Work out the finished part from the listing and answer in its coordinate system (mm). Face numbers are marked on the shaded views. A direction names the side the tool comes from. Round coordinates to 2 decimals unless told otherwise and drop trailing zeros. Write each loop counter-clockwise with the first axis right and the second up, starting at its lowest first coordinate (ties: lowest second). Pieces come first, ordered by that corner, then holes. Notation, with made-up numbers: (80, 82) - (105, 82) arc R25 cw to (105, 119) - close; hole circle Ø7 at (-16.5, 29). An arc over 180 degrees is marked (long way). Answer as a JSON object with one key per item and string values.
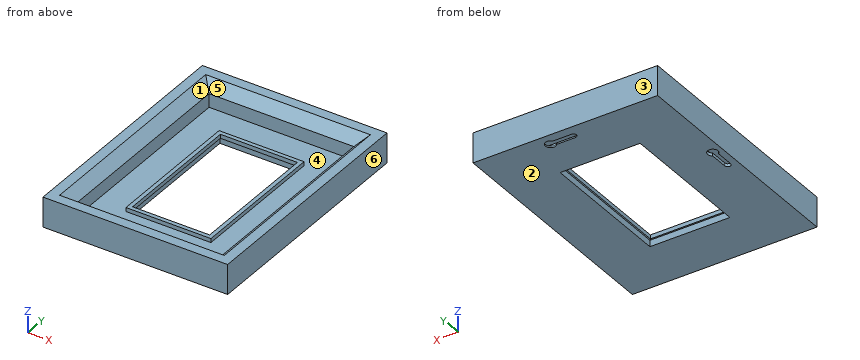
```python
from build123d import *

# Parameters (mm, degrees)
SKETCH_W             = 185.32
SKETCH_H             = 240.5
PAD_DEPTH            = 30
SKETCH003_W          = 145.32
SKETCH003_H          = 200.5
POCKET_DEPTH         = 23.6
SKETCH004_W          = 80.32
SKETCH004_H          = 135.5
POCKET001_DEPTH      = 6.4
POCKET002_DEPTH      = 3
SKETCH006_W          = 14
SKETCH006_H          = 3
POCKET003_DEPTH      = 30
POCKET004_DEPTH      = 1.5
SKETCH008_W          = 12
SKETCH008_H          = 2.4244
POCKET005_DEPTH      = 30
SKETCH009_W          = 85.32
SKETCH009_H          = 140.5
PAD001_DEPTH         = 4
SKETCH010_W          = 77.32
SKETCH010_H          = 132.5
POCKET006_DEPTH      = 0.001
POCKET006_DEPTH_BACK = -30.001
CHAMFER_SIZE         = 10


with BuildPart() as part:
    # Sketch → Pad (new body)
    with BuildSketch(Plane.XY):
        Rectangle(SKETCH_W, SKETCH_H)
    extrude(amount=PAD_DEPTH)

    # Sketch003 → Pocket (cut)
    with BuildSketch(Plane.XY.offset(30)):
        Rectangle(SKETCH003_W, SKETCH003_H)
    extrude(amount=-POCKET_DEPTH, mode=Mode.SUBTRACT)

    # Sketch004 → Pocket001 (cut)
    with BuildSketch(Plane.XY.offset(6.4)):
        Rectangle(SKETCH004_W, SKETCH004_H)
    extrude(amount=-POCKET001_DEPTH, mode=Mode.SUBTRACT)

    # Sketch005 → Pocket002 (cut)
    with BuildSketch(Plane.XY):
        with BuildLine():
            ThreePointArc((-85.97, 0), (-82.985, -2.985), (-80, 0))
            Line((-80, 0), (-80, 18.025988))
            ThreePointArc((-80, 18.025988), (-82.985, 27.495), (-85.97, 18.025988))
            Line((-85.97, 18.025988), (-85.97, 0))
        make_face()
    extrude(amount=POCKET002_DEPTH, mode=Mode.SUBTRACT)

    # Sketch006 → Pocket003 (cut, symmetric)
    with BuildSketch(Plane.XZ):
        with Locations((-83, 4.48)):
            Rectangle(SKETCH006_W, SKETCH006_H)
    extrude(amount=POCKET003_DEPTH, both=True, mode=Mode.SUBTRACT)

    # Sketch007 → Pocket004 (cut, symmetric)
    with BuildSketch(Plane.XY):
        with BuildLine():
            ThreePointArc((0, 110.985), (-2.985, 108), (0, 105.015))
            Line((0, 105.015), (18.705988, 105.015))
            ThreePointArc((18.705988, 105.015), (28.175, 108), (18.705988, 110.985))
            Line((18.705988, 110.985), (0, 110.985))
        make_face()
    extrude(amount=POCKET004_DEPTH, both=True, mode=Mode.SUBTRACT)

    # Sketch008 → Pocket005 (cut, symmetric)
    with BuildSketch(Plane.YZ):
        with Locations((108, 2.7105)):
            Rectangle(SKETCH008_W, SKETCH008_H)
    extrude(amount=POCKET005_DEPTH, both=True, mode=Mode.SUBTRACT)

    # Sketch009 → Pad001 (join)
    with BuildSketch(Plane.XY.offset(6.4)):
        Rectangle(SKETCH009_W, SKETCH009_H)
    extrude(amount=PAD001_DEPTH)

    # Sketch010 → Pocket006 (cut, two sides)
    with BuildSketch(Plane.XY) as pocket006_sk:
        Rectangle(SKETCH010_W, SKETCH010_H)
    extrude(amount=-POCKET006_DEPTH, mode=Mode.SUBTRACT)
    extrude(pocket006_sk.sketch, amount=-POCKET006_DEPTH_BACK, mode=Mode.SUBTRACT)

    # Chamfer
    chamfer_edges = [part.edges().sort_by_distance(p)[0] for p in [
        (-72.66, 0, 30),
        (0, 100.25, 30),
        (72.66, 0, 30),
        (0, -100.25, 30),
    ]]
    chamfer(chamfer_edges, length=CHAMFER_SIZE)


solid = part.part
```
Item 1: A cutting plane is placed at D-D (z = 26). Write down the section's boundary in (x, y).
Results found:
{"outline": "(-92.66, -120.25) - (92.66, -120.25) - (92.66, 120.25) - (-92.66, 120.25) - close; hole (-78.66, -106.25) - (78.66, -106.25) - (78.66, 106.25) - (-78.66, 106.25) - close"}
Item 2: Determine the mould class of the marked faces 3, 4, 5 and 6 for opening direction Y: pulls with the +Y half, pulls with the -Y half, needs draft (parallel to the pull), parting line crosses it, or undercut.
Results found:
{"face 3": "pulls with the +Y half", "face 4": "undercut", "face 5": "undercut", "face 6": "needs draft"}
Item 3: For the marked faces 1 and 2, determine the directions among +Z, -Z, +X, -X, +Y, -Y from which every point of the face is accessible in a straight line to the end or side of a thin tool.
Results found:
{"face 1": "+Z", "face 2": "-Z, +X, -X, +Y, -Y"}
Item 4: Consider line 1 along Y through (x, z) = (22.97, 1.2) (3 decimals); line 2 along X through (y, z) = (-30.5, 7.5); line 3 along X through (y, z) = (22, 1). Determine where each line is inside the solid, lowest interval first.
Results found:
{"line 1": "-120.25 to -67.75, 67.75 to 102.795, 113.205 to 120.25", "line 2": "-92.66 to -72.66, -42.66 to -38.66, 38.66 to 42.66, 72.66 to 92.66", "line 3": "-92.66 to -88.18, -77.79 to -40.16, 40.16 to 92.66"}
Item 5: A cutting plane is placed at A-A (x = -26). Write down the section's boundary in (y, z).
Results found:
{"outline": "(-120.25, 0) - (-67.75, 0) - (-67.75, 6.4) - (-66.25, 6.4) - (-66.25, 10.4) - (-70.25, 10.4) - (-70.25, 6.4) - (-100.25, 6.4) - (-100.25, 20) - (-110.25, 30) - (-120.25, 30) - close; (66.25, 6.4) - (67.75, 6.4) - (67.75, 0) - (120.25, 0) - (120.25, 30) - (110.25, 30) - (100.25, 20) - (100.25, 6.4) - (70.25, 6.4) - (70.25, 10.4) - (66.25, 10.4) - close; hole (102, 1.5) - (114, 1.5) - (114, 3.92) - (102, 3.92) - close"}
